from build123d import *

# Parameters (mm, degrees)
F0_W     = 51
F0_H     = 170
F0_R     = 1.5
F1_DEPTH = 3
F2_DEPTH = 3
F3_DEPTH = 15


with BuildPart() as f1:
    # F0 (on Front) → F1 (new body)
    with BuildSketch(Plane.XZ):
        with Locations((-25.5, 85)):
            Rectangle(F0_W, F0_H)
        with Locations((-29, 14)):
            Circle(F0_R, mode=Mode.SUBTRACT)
        with Locations((-29, 142)):
            Circle(F0_R, mode=Mode.SUBTRACT)
    extrude(amount=F1_DEPTH)

    # F0 (on Front) → F2 (join)
    with BuildSketch(Plane.XZ):
        Polygon((0, 170), (0, 0), (-51, 0), (-51, -5), (0, -5), (5, -5), (5, 170), align=None)
    extrude(amount=F2_DEPTH)

    # F0 (on Front) → F3 (join)
    with BuildSketch(Plane.XZ):
        Polygon((0, 170), (0, 0), (-51, 0), (-51, -5), (0, -5), (5, -5), (5, 170), align=None)
    extrude(amount=-F3_DEPTH)


solid = f1.part
Can you work these out from the model? Positions are in its coordinate system, mm. A direction names the side the tool comes from. Coordinates: 2 decimals unless noted, no trailing zeros. Write each loop counter-clockwise with the first axis right and the second up, starting at its lowest first coordinate (ties: lowest second). Pieces come first, ordered by that corner, then holes. Notation, with made-up numbers: (7, 21) -> (23, 21) arc R30 ccw to (23, 59) -> close; hole circle Ø6 at (-26, -32.5). An arc over 180 degrees is marked (long way). Answer as CSV lines item,"result".
1) If we mould it in two halves opening along Z, with no side actions, what happens to faces 1 (the flat face through (0, 7, 86)), 2 (the flat face through (-25, 7, 0)), 3 (the cylindrical face through (-29.195, -1.479, 143.487))? For each: +Z half, -Z half, draft (parallel to the pull), parting line (faces both ways), or undercut.
Check result:
face 1,"draft"
face 2,"+Z half"
face 3,"undercut"
2) If we section it at B-B on z = 142: Please give me the cut outline in (x, y).
Check result:
outline,"(-51, -3) -> (-30.5, -3) -> (-30.5, 0) -> (-51, 0) -> close; (-27.5, -3) -> (5, -3) -> (5, 15) -> (0, 15) -> (0, 0) -> (-27.5, 0) -> close"
3) On a 3-axis mill with a long thin cutter (end or side, diameter ignored), from which of +Z, -Z, +X, -X, +Y, -Y can I reach the whole of each face in a straight line? I mean faces 4 (the flat face through (-26, 0, 86)), 5 (the flat face through (-51, -1, 70)). Say none if no direction works.
Check result:
face 4,"+Z, -X, +Y"
face 5,"+Z, -Z, -X, +Y, -Y"
4) Will these pins go through, and if not, where does the flat tip stop? P1, Ø10, axis at x = -27.5, y = 7, coming from the +Z side; P2, Ø10, axis at x = -12, z = 72, coming from the +Y side; P3, Ø1, axis at y = 10, z = 18.5, coming from the -X side; P4, Ø1.8, axis at x = -29, z = 14, coming from the -Y side.
Check result:
P1,"z = 0"
P2,"y = 0"
P3,"x = 0"
P4,"through"
5) If we section it at C-C on z = 124.5: Please give me the cut outline in (x, y), then the cut area to 3 significant figures.
Check result:
outline,"(-51, -3) -> (5, -3) -> (5, 15) -> (0, 15) -> (0, 0) -> (-51, 0) -> close"
area,"243 mm²"
6) If we section it at D-D on y = 13.5: Please give me the cut outline in (x, z).
Check result:
outline,"(-51, -5) -> (5, -5) -> (5, 170) -> (0, 170) -> (0, 0) -> (-51, 0) -> close"
7) If we section it at A-A on x = -29: Please give me the cut outline in (y, z).
Check result:
outline,"(-3, -5) -> (15, -5) -> (15, 0) -> (0, 0) -> (0, 12.5) -> (-3, 12.5) -> close; (-3, 15.5) -> (0, 15.5) -> (0, 140.5) -> (-3, 140.5) -> close; (-3, 143.5) -> (0, 143.5) -> (0, 170) -> (-3, 170) -> close"
8) If I drill on line 1 (Z direction, x = -29, y = -1.6); line 2 (X direction, y = -1.2, z = 142); line 3 (X direction, y = 8.25, z = 15.5), over which ranges is the centre line in solid material (lowest first)? Write a range as from..to.
Check result:
line 1,"-5..12.5, 15.5..140.5, 143.5..170"
line 2,"-51..-30.5, -27.5..5"
line 3,"0..5"
